from build123d import *

# Parameters (mm, degrees)
CYLINDER007_R            = 1.8
CYLINDER007_DEPTH        = 10
ARRAY004_X_COUNT         = 2
ARRAY004_X_PITCH         = 20
ARRAY004_Y_COUNT         = 2
ARRAY004_Y_PITCH         = 20
ARRAY004_PLACEMENT_ANGLE = 90
BOX021_W                 = 32
BOX021_H                 = 3
BOX021_DEPTH             = 38
FILLET_R                 = 8


with BuildPart() as top_bolt_hole_array:
    # Cylinder007 → Cylinder007 (new body)
    with BuildSketch(Plane.XY):
        Circle(CYLINDER007_R)
    extrude(amount=CYLINDER007_DEPTH)

    # Array004 X: top bolt hole array ×2


with BuildPart() as top_bolt_hole_array_1:
    add(top_bolt_hole_array.part)
    with Locations(*[(i * ARRAY004_X_PITCH, 0, 0) for i in range(1, ARRAY004_X_COUNT)]):
        add(top_bolt_hole_array.part)

    # Array004 Y: top bolt hole array ×2


with BuildPart() as top_bolt_hole_array_2:
    add(top_bolt_hole_array_1.part)
    with Locations(*[(0, i * ARRAY004_Y_PITCH, 0) for i in range(1, ARRAY004_Y_COUNT)]):
        add(top_bolt_hole_array_1.part)


with BuildPart() as top_bolt_hole_array_3:
    # Array004 placement: moved
    add(top_bolt_hole_array_2.part.moved(Location((24, 88, 16))).rotate(Axis((24, 88, 16), (1, 0, 0)), ARRAY004_PLACEMENT_ANGLE))


with BuildPart() as cut001005:
    # Box021 → Box021 (new body)
    with BuildSketch(Plane(origin=(18, 82, 9.5), x_dir=(1, 0, 0), z_dir=(0, 0, 1))):
        with Locations((16, 1.5)):
            Rectangle(BOX021_W, BOX021_H)
    extrude(amount=BOX021_DEPTH)

    # Fillet
    fillet_edges = [cut001005.edges().sort_by_distance(p)[0] for p in [
        (18, 83.5, 9.5),
        (50, 83.5, 9.5),
    ]]
    fillet(fillet_edges, radius=FILLET_R)

    # Cut001005: cut top bolt hole array
    add(top_bolt_hole_array_3.part, mode=Mode.SUBTRACT)


solid = cut001005.part
Verification items for the finished model (mm, model axes). Give positions to 0.01 mm unless a question says otherwise; leave off trailing zeros. Loops run counter-clockwise (first coordinate to the right, second up) from the corner with the lowest first, then second, coordinate; pieces in that order, holes last. Notation, with made-up numbers: (-12.75, 68) - (45.25, 68) arc R3 ccw to (45.25, 72) - close; hole circle Ø1 at (-8, 82). An arc over 180 degrees is marked (long way). Write item = value, one per line. Start each with the question number.
Q1. Cross-section at C-C, the plane y = 84.2. Enter the section's corners in (x, z).
Q2. Thickness scan on line 1 (X direction, y = 82.7, z = 36); line 2 (Z direction, x = 44, y = 83.65); line 3 (X direction, y = 83.4, z = 16). Record the ranges inside material, lowest first.
Q3. Depth check by flat-ended pin: P1, Ø2, axis at x = 44, z = 36, coming from the +Y side; P2, Ø1.5, axis at x = 46.5, y = 83, coming from the -Z side. Enter the tip coordinate at first touch or a pass-through.
Q4. Mould release check, pull along Z, two halves, no side actions. Record for faces 1 (the face through (34, 84, 47.5)), 2 (the face through (25.717, 83.521, 36.541)), 3 (the face through (47.719, 83.521, 11.906)): released by +Z, released by -Z, zero draft, split by the parting line, or undercut.
Q5. Cross-section at A-A, the plane z = 36. Enter the section's corners in (x, y), and give its area (3 significant figures).
Q6. Cross-section at D-D, the plane x = 47. Enter the section's corners in (y, z) (3 decimals), and give its area (3 significant figures).
Q7. Cross-section at B-B, the plane x = 24. Enter the section's corners in (y, z).
Answer key:
q1.outline = (18, 17.5) arc R8 ccw to (26, 9.5) - (42, 9.5) arc R8 ccw to (50, 17.5) - (50, 47.5) - (18, 47.5) - close; hole circle Ø3.6 at (24, 16); hole circle Ø3.6 at (24, 36); hole circle Ø3.6 at (44, 16); hole circle Ø3.6 at (44, 36)
q2.line_1 = 18 to 22.2, 25.8 to 42.2, 45.8 to 50
q2.line_2 = 9.75 to 14.2, 17.8 to 34.2, 37.8 to 47.5
q2.line_3 = 18.14 to 22.2, 25.8 to 42.2, 45.8 to 49.86
q3.P1 = through
q3.P2 = 10.43
q4.face_1 = released by +Z
q4.face_2 = undercut
q4.face_3 = released by -Z
q5.outline = (18, 82) - (22.2, 82) - (22.2, 85) - (18, 85) - close; (25.8, 82) - (42.2, 82) - (42.2, 85) - (25.8, 85) - close; (45.8, 82) - (50, 82) - (50, 85) - (45.8, 85) - close
q5.area = 74.4 mm^2
q6.outline = (82, 11.255) - (85, 11.255) - (85, 47.5) - (82, 47.5) - close
q6.area = 109 mm^2
q7.outline = (82, 9.75) - (85, 9.75) - (85, 14.2) - (82, 14.2) - close; (82, 17.8) - (85, 17.8) - (85, 34.2) - (82, 34.2) - close; (82, 37.8) - (85, 37.8) - (85, 47.5) - (82, 47.5) - close
